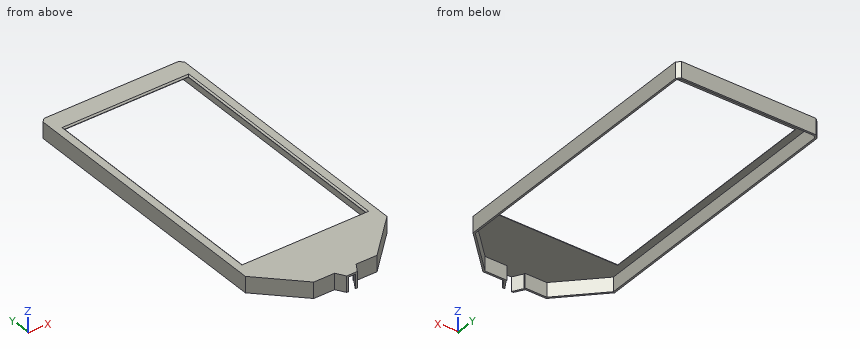
Autodesk Inventor part; units mm, degrees
ref_plane "YZ Plane" through (0, 0, 0) normal (1, 0, 0) x (0, 1, 0)
ref_plane "XZ Plane" through (0, 0, 0) normal (0, 1, 0) x (-1, 0, 0)
ref_plane "XY Plane" through (0, 0, 0) normal (0, 0, 1) x (1, 0, 0)
sketch "Boceto1" plane through (0, 0, 0) normal (0, 0, 1) x (1, 0, 0)
  line L0 (-39.75, -78.25) -> (39.75, -78.25)
  line L1 (39.75, -78.25) -> (39.75, 78.25)
  line L2 (39.75, 78.25) -> (-39.75, 78.25)
  line L3 (-39.75, 78.25) -> (-39.75, -78.25)
  line L4 (-39.75, -78.25) -> (39.75, 78.25) construction
  line L5 (39.75, -78.25) -> (-39.75, 78.25) construction
  point P0 (0, 0)
  dimension "d0" = 79.5
  dimension "d1" = 156.5
extrude "Extrusión1" add sketch "Boceto1" along normal blind 9
sketch "Boceto2" plane through (0, 0, 9) normal (0, 0, 1) x (1, 0, 0)
  line L0 (-39.75, -78.25) -> (39.75, -78.25)
  line L1 (-6, -78.25) -> (-6, -98.25)
  line L2 (-6, -98.25) -> (-3, -103.25)
  line L3 (-3, -103.25) -> (3, -103.25)
  line L4 (3, -103.25) -> (6, -98.25)
  line L5 (6, -98.25) -> (6, -78.25)
  point P0 (0, 0)
  point P1 (6, -88.25)
  point P2 (-6, -88.25)
  point P3 (0, -78.25)
  point P4 (0, -103.25)
  point P5 (0, -78.25)
  dimension "d4" = 12
  dimension "d5" = 6
  dimension "d6" = 20
  dimension "d7" = 5
  dimension "d8" = 6
extrude "Extrusión2" add sketch "Boceto2" against normal up to surface (9 mm away)
chamfer "Chaflán2" distance 2 angle 45 4 edges at (-39.75, -78.25, 4.5) (-39.75, 78.25, 4.5) (39.75, -78.25, 4.5) (39.75, 78.25, 4.5)
shell "Vaciado1" thickness 1 removed faces 2 at (-2, 24.75, 0) at (-1, -103.25, 6)
sketch "Boceto3" plane through (0, 0, 9) normal (0, 0, 1) x (1, 0, 0)
  line L0 (-34.75, 66.75) -> (34.75, 66.75)
  line L1 (34.75, 66.75) -> (34.75, -67.25)
  line L2 (34.75, -67.25) -> (-34.75, -67.25)
  line L3 (-34.75, -67.25) -> (-34.75, 66.75)
  line L4 (-34.75, 66.75) -> (34.75, -67.25) construction
  line L5 (34.75, 66.75) -> (-34.75, -67.25) construction
  line L6 (37.3358, 77.25) -> (38.75, 75.8358)
  line L7 (38.75, -75.8358) -> (38.75, 75.8358)
  line L8 (38.75, -75.8358) -> (37.3358, -77.25)
  line L9 (5, -77.25) -> (37.3358, -77.25)
  line L10 (5, -97.973) -> (5, -77.25)
  line L11 (1.8338, -103.25) -> (5, -97.973)
  line L12 (-1.8338, -103.25) -> (1.8338, -103.25)
  line L13 (-5, -97.973) -> (-1.8338, -103.25)
  line L14 (-5, -77.25) -> (-5, -97.973)
  line L15 (-37.3358, -77.25) -> (-5, -77.25)
  line L16 (-37.3358, -77.25) -> (-38.75, -75.8358)
  line L17 (-38.75, 75.8358) -> (-38.75, -75.8358)
  line L18 (-38.75, 75.8358) -> (-37.3358, 77.25)
  line L19 (37.3358, 77.25) -> (-37.3358, 77.25)
  point P0 (0, 0)
  point P1 (0, -0.25)
  dimension "d18" = 4
  dimension "d19" = 4
  dimension "d20" = 10.5
  dimension "d21" = 10
extrude "Extrusión3" cut sketch "Boceto3" against normal blind 10 contours L0 L1 L2 L3
chamfer "Chaflán3" distance 0.8 angle 45 4 edges at (0, 66.75, 9) (34.75, -0.25, 9) (0, -67.25, 9) (-34.75, -0.25, 9)
move faces "Desplazar1" translate (0, -20, 0) faces at (-27.1667, -78.25, 3) (16.5833, -78.25, 3) (-26.5572, -77.25, 2.6667) (26.5572, -77.25, 5.3333)
properties part number "BiselTelefono"
The listing builds one solid part. Answer for the finished solid, in the listing's coordinates (mm). Give positions to 0.01 mm unless a question says otherwise; leave off trailing zeros. Order: outer loops, then holes, each group sorted by start corner. A loop starts at its lowest first (then second) coordinate and runs counter-clockwise, first axis right, second up. Notation, with made-up numbers: (36.25, 73.5) - (40.25, 73.5) arc R19 cw to (40.25, 94.5) - close; hole circle Ø1 at (-16.75, 77). An arc over 180 degrees is marked (long way). Answer in a Markdown table with one row per item. Add a question column.
Q1. The part is cut by section D-D (y = -88.5). Determine the outline of the cut face in (x, z).
Q2. Find the intervals of material crossed by line 1 along X through (y, z) = (-68.5, 5.75); line 2 along Y through (x, z) = (-11, 3.25); line 3 along X through (y, z) = (-88.5, 6.25), in increasing order. Write a range as [from, to].
Q3. The part is cut by section C-C (z = 3.5). Determine the outline of the cut face in (x, y), then the cut area to 3 significant figures.
Q4. The part is cut by section B-B (x = -32.5). Determine the outline of the cut face in (y, z), then the cut area to 3 significant figures.
Q5. The part is cut by section A-A (y = -6). Determine the outline of the cut face in (x, z).
Q6. Given P1, Ø0.8, axis at y = -97.5, z = 3, coming from the +X side; P2, Ø1, axis at x = -5, z = 4.5, coming from the -Y side; P3, Ø2.5, axis at x = 1, z = 4, coming from the -Y side; P4, Ø0.6, axis at y = -97.5, z = 4.5, coming from the -X side, each flat-ended and moving along its own axis, determine where each tip first touches the part or whether it passes through.
Determined:
| question | item | result |
|---|---|---|
| 1 | outline | (-27.5, 0) - (-26.09, 0) - (-26.09, 8) - (26.09, 8) - (26.09, 0) - (27.5, 0) - (27.5, 9) - (-27.5, 9) - close |
| 2 | line 1 | x = [-39.75, -38.75], [38.75, 39.75] |
| 2 | line 2 | y = [-98.25, -97.25], [77.25, 78.25] |
| 2 | line 3 | x = [-27.5, -26.09], [26.09, 27.5] |
| 3 | outline | (-39.75, -76.25) - (-17.75, -98.25) - (-6, -98.25) - (-3, -103.25) - (-1.83, -103.25) - (-5, -97.97) - (-5, -97.25) - (-17.34, -97.25) - (-38.75, -75.84) - (-38.75, 75.84) - (-37.34, 77.25) - (37.34, 77.25) - (38.75, 75.84) - (38.75, -75.84) - (17.34, -97.25) - (5, -97.25) - (5, -97.97) - (1.83, -103.25) - (3, -103.25) - (6, -98.25) - (17.75, -98.25) - (39.75, -76.25) - (39.75, 76.25) - (37.75, 78.25) - (-37.75, 78.25) - (-39.75, 76.25) - close |
| 3 | area | 482 mm² |
| 4 | outline | (-83.5, 0) - (-82.09, 0) - (-82.09, 8) - (-67.25, 8) - (-67.25, 8.2) - (-68.05, 9) - (-83.5, 9) - close; (66.75, 8) - (77.25, 8) - (77.25, 0) - (78.25, 0) - (78.25, 9) - (67.55, 9) - (66.75, 8.2) - close |
| 4 | area | 46.4 mm² |
| 5 | outline | (-39.75, 0) - (-38.75, 0) - (-38.75, 8) - (-34.75, 8) - (-34.75, 8.2) - (-35.55, 9) - (-39.75, 9) - close; (34.75, 8) - (38.75, 8) - (38.75, 0) - (39.75, 0) - (39.75, 9) - (35.55, 9) - (34.75, 8.2) - close |
| 6 | P1 | stops at x = 18.9 |
| 6 | P2 | stops at y = -100.75 |
| 6 | P3 | stops at y = -103.25 |
| 6 | P4 | stops at x = -18.8 |
